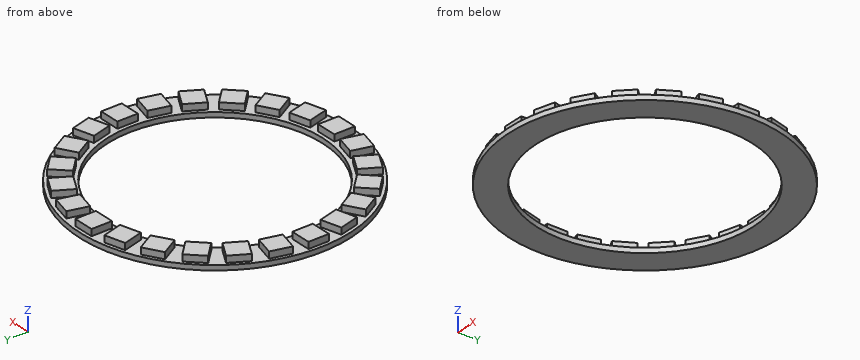
Autodesk Fusion 360 part; units mm, degrees
sketch "Sketch1" plane through (0, 0, 0) normal (0, 0, 1) x (1, 0, 0)
  circle A0 centre (0, 0) radius 33
  circle A1 centre (0, 0) radius 26.25
  line L0 (0.0215, 33) -> (0.0215, 26.25) construction
  line L1 (2.5215, 27.125) -> (-2.4785, 27.125)
  line L2 (-2.4785, 27.125) -> (-2.4785, 32.125)
  line L3 (-2.4785, 32.125) -> (2.5215, 32.125)
  line L4 (2.5215, 32.125) -> (2.5215, 27.125)
  line L5 (2.5215, 27.125) -> (-2.4785, 32.125) construction
  line L6 (-2.4785, 27.125) -> (2.5215, 32.125) construction
  line L7 (-10.7086, 30.3889) -> (-5.879, 31.683)
  line L8 (-5.879, 31.683) -> (-4.5849, 26.8533)
  line L9 (-4.5849, 26.8533) -> (-9.4145, 25.5592)
  line L10 (-9.4145, 25.5592) -> (-10.7086, 30.3889)
  line L11 (-18.2089, 26.5818) -> (-13.8788, 29.0818)
  line L12 (-13.8788, 29.0818) -> (-11.3788, 24.7517)
  line L13 (-11.3788, 24.7517) -> (-15.7089, 22.2517)
  line L14 (-15.7089, 22.2517) -> (-18.2089, 26.5818)
  line L15 (-24.4684, 20.9632) -> (-20.9328, 24.4988)
  line L16 (-20.9328, 24.4988) -> (-17.3973, 20.9632)
  line L17 (-17.3973, 20.9632) -> (-20.9328, 17.4277)
  line L18 (-20.9328, 17.4277) -> (-24.4684, 20.9632)
  line L19 (-29.0603, 13.9161) -> (-26.5603, 18.2462)
  line L20 (-26.5603, 18.2462) -> (-22.2302, 15.7462)
  line L21 (-22.2302, 15.7462) -> (-24.7302, 11.4161)
  line L22 (-24.7302, 11.4161) -> (-29.0603, 13.9161)
  line L23 (-31.6718, 5.9205) -> (-30.3777, 10.7501)
  line L24 (-30.3777, 10.7501) -> (-25.5481, 9.456)
  line L25 (-25.5481, 9.456) -> (-26.8422, 4.6264)
  line L26 (-26.8422, 4.6264) -> (-31.6718, 5.9205)
  line L27 (-32.125, -2.4785) -> (-32.125, 2.5215)
  line L28 (-32.125, 2.5215) -> (-27.125, 2.5215)
  line L29 (-27.125, 2.5215) -> (-27.125, -2.4785)
  line L30 (-27.125, -2.4785) -> (-32.125, -2.4785)
  line L31 (-30.3889, -10.7086) -> (-31.683, -5.879)
  line L32 (-31.683, -5.879) -> (-26.8533, -4.5849)
  line L33 (-26.8533, -4.5849) -> (-25.5592, -9.4145)
  line L34 (-25.5592, -9.4145) -> (-30.3889, -10.7086)
  line L35 (-26.5818, -18.2089) -> (-29.0818, -13.8788)
  line L36 (-29.0818, -13.8788) -> (-24.7517, -11.3788)
  line L37 (-24.7517, -11.3788) -> (-22.2517, -15.7089)
  line L38 (-22.2517, -15.7089) -> (-26.5818, -18.2089)
  line L39 (-20.9632, -24.4684) -> (-24.4988, -20.9328)
  line L40 (-24.4988, -20.9328) -> (-20.9632, -17.3973)
  line L41 (-20.9632, -17.3973) -> (-17.4277, -20.9328)
  line L42 (-17.4277, -20.9328) -> (-20.9632, -24.4684)
  line L43 (-13.9161, -29.0603) -> (-18.2462, -26.5603)
  line L44 (-18.2462, -26.5603) -> (-15.7462, -22.2302)
  line L45 (-15.7462, -22.2302) -> (-11.4161, -24.7302)
  line L46 (-11.4161, -24.7302) -> (-13.9161, -29.0603)
  line L47 (-5.9205, -31.6718) -> (-10.7501, -30.3777)
  line L48 (-10.7501, -30.3777) -> (-9.456, -25.5481)
  line L49 (-9.456, -25.5481) -> (-4.6264, -26.8422)
  line L50 (-4.6264, -26.8422) -> (-5.9205, -31.6718)
  line L51 (2.4785, -32.125) -> (-2.5215, -32.125)
  line L52 (-2.5215, -32.125) -> (-2.5215, -27.125)
  line L53 (-2.5215, -27.125) -> (2.4785, -27.125)
  line L54 (2.4785, -27.125) -> (2.4785, -32.125)
  line L55 (10.7086, -30.3889) -> (5.879, -31.683)
  line L56 (5.879, -31.683) -> (4.5849, -26.8533)
  line L57 (4.5849, -26.8533) -> (9.4145, -25.5592)
  line L58 (9.4145, -25.5592) -> (10.7086, -30.3889)
  line L59 (18.2089, -26.5818) -> (13.8788, -29.0818)
  line L60 (13.8788, -29.0818) -> (11.3788, -24.7517)
  line L61 (11.3788, -24.7517) -> (15.7089, -22.2517)
  line L62 (15.7089, -22.2517) -> (18.2089, -26.5818)
  line L63 (24.4684, -20.9632) -> (20.9328, -24.4988)
  line L64 (20.9328, -24.4988) -> (17.3973, -20.9632)
  line L65 (17.3973, -20.9632) -> (20.9328, -17.4277)
  line L66 (20.9328, -17.4277) -> (24.4684, -20.9632)
  line L67 (29.0603, -13.9161) -> (26.5603, -18.2462)
  line L68 (26.5603, -18.2462) -> (22.2302, -15.7462)
  line L69 (22.2302, -15.7462) -> (24.7302, -11.4161)
  line L70 (24.7302, -11.4161) -> (29.0603, -13.9161)
  line L71 (31.6718, -5.9205) -> (30.3777, -10.7501)
  line L72 (30.3777, -10.7501) -> (25.5481, -9.456)
  line L73 (25.5481, -9.456) -> (26.8422, -4.6264)
  line L74 (26.8422, -4.6264) -> (31.6718, -5.9205)
  line L75 (32.125, 2.4785) -> (32.125, -2.5215)
  line L76 (32.125, -2.5215) -> (27.125, -2.5215)
  line L77 (27.125, -2.5215) -> (27.125, 2.4785)
  line L78 (27.125, 2.4785) -> (32.125, 2.4785)
  line L79 (30.3889, 10.7086) -> (31.683, 5.879)
  line L80 (31.683, 5.879) -> (26.8533, 4.5849)
  line L81 (26.8533, 4.5849) -> (25.5592, 9.4145)
  line L82 (25.5592, 9.4145) -> (30.3889, 10.7086)
  line L83 (26.5818, 18.2089) -> (29.0818, 13.8788)
  line L84 (29.0818, 13.8788) -> (24.7517, 11.3788)
  line L85 (24.7517, 11.3788) -> (22.2517, 15.7089)
  line L86 (22.2517, 15.7089) -> (26.5818, 18.2089)
  line L87 (20.9632, 24.4684) -> (24.4988, 20.9328)
  line L88 (24.4988, 20.9328) -> (20.9632, 17.3973)
  line L89 (20.9632, 17.3973) -> (17.4277, 20.9328)
  line L90 (17.4277, 20.9328) -> (20.9632, 24.4684)
  line L91 (13.9161, 29.0603) -> (18.2462, 26.5603)
  line L92 (18.2462, 26.5603) -> (15.7462, 22.2302)
  line L93 (15.7462, 22.2302) -> (11.4161, 24.7302)
  line L94 (11.4161, 24.7302) -> (13.9161, 29.0603)
  line L95 (5.9205, 31.6718) -> (10.7501, 30.3777)
  line L96 (10.7501, 30.3777) -> (9.456, 25.5481)
  line L97 (9.456, 25.5481) -> (4.6264, 26.8422)
  line L98 (4.6264, 26.8422) -> (5.9205, 31.6718)
  point P0 (0.0215, 29.625)
  dimension "d1" = 66
  dimension "d2" = 52.5
  dimension "d3" = 5
  dimension "d4" = 5
  dimension "d6" = 360
extrude "Extrude1" add sketch "Sketch1" against normal blind 1.2 contours A0 | L1 L2 L3 L4 | L7 L8 L9 L10 | L11 L12 L13 L14 | L15 L16 L17 L18 | L19 L20 L21 L22 | L23 L24 L25 L26 | L27 L28 L29 L30 | L31 L32 L33 L34 | L35 L36 L37 L38 | L39 L40 L41 L42 | L43 L44 L45 L46 | L47 L48 L49 L50 | L51 L52 L53 L54 | L55 L56 L57 L58 | L59 L60 L61 L62 | L63 L64 L65 L66 | L67 L68 L69 L70 | L71 L72 L73 L74 | L75 L76 L77 L78 | L79 L80 L81 L82 | L83 L84 L85 L86 | L87 L88 L89 L90 | L91 L92 L93 L94 | L95 L96 L97 L98
extrude "Extrude2" add sketch "Sketch1" along normal blind 1.6 contours L1 L2 L3 L4 | L7 L8 L9 L10 | L11 L12 L13 L14 | L15 L16 L17 L18 | L19 L20 L21 L22 | L23 L24 L25 L26 | L27 L28 L29 L30 | L31 L32 L33 L34 | L35 L36 L37 L38 | L39 L40 L41 L42 | L43 L44 L45 L46 | L47 L48 L49 L50 | L51 L52 L53 L54 | L55 L56 L57 L58 | L59 L60 L61 L62 | L63 L64 L65 L66 | L67 L68 L69 L70 | L71 L72 L73 L74 | L75 L76 L77 L78 | L79 L80 L81 L82 | L83 L84 L85 L86 | L87 L88 L89 L90 | L91 L92 L93 L94 | L95 L96 L97 L98
The listing builds one solid part. Answer for the finished solid, in the listing's coordinates (mm). Round coordinates to 2 decimals unless told otherwise and drop trailing zeros. Order: outer loops, then holes, each group sorted by start corner. A loop starts at its lowest first (then second) coordinate and runs counter-clockwise, first axis right, second up. Notation, with made-up numbers: (10, -28.5) -> (14, -28.5) arc R8 ccw to (14, -21.5) -> close; hole circle Ø10 at (14.25, 7.25). An arc over 180 degrees is marked (long way). Answer as CSV lines item,"result".
Q1. A cutting plane is placed at C-C on z = 0.45. Give the number of separate pieces and of enclosed holes in the cut face, plus the area to 3 significant figures.
Computed values:
separate pieces,"24"
enclosed holes,"0"
area,"600 mm^2"
Q2. A cutting plane is placed at A-A on x = 0. Determine the outline of the cut face in (y, z) (3 decimals), plus the area to 3 significant figures.
Computed values:
outline,"(-33, -1.2) -> (-26.25, -1.2) -> (-26.25, 0) -> (-27.125, 0) -> (-27.125, 1.6) -> (-32.125, 1.6) -> (-32.125, 0) -> (-33, 0) -> close; (26.25, -1.2) -> (33, -1.2) -> (33, 0) -> (32.125, 0) -> (32.125, 1.6) -> (27.125, 1.6) -> (27.125, 0) -> (26.25, 0) -> close"
area,"32.2 mm^2"
Q3. Consider line 1 (Y direction, x = 0, z = -0.75); line 2 (Y direction, x = 28, z = 1.3); line 3 (X direction, y = -18.5, z = 1.05). Determine where each line is inside the solid, lowest interval first. Write a range as from..to.
Computed values:
line 1,"y = -33..-26.25, 26.25..33"
line 2,"y = -15.75..-13.3, -10.11..-4.94, -2.52..2.48, 4.89..10.07, 13.25..15.75"
line 3,"x = -22.07..-19.86, 19.86..22.01"
Q4. Given pin 1 (0.5 mm diameter, centred on x = 0, z = 0.5, fed in from +Y) (3 decimals); pin 2 (0.8 mm diameter, centred on x = -29, z = 1, fed in from +Y); pin 3 (0.8 mm diameter, centred on y = 29, z = 0.5, fed in from -X), each flat-ended and moving along its own axis, determine where each tip first touches the part or whether it passes through.
Computed values:
pin 1,"stops at y = 32.125"
pin 2,"stops at y = 14.71"
pin 3,"stops at x = -14.71"
